from build123d import *

# Parameters (mm, degrees)
SKIZZE1_R                        = 22.5
SEITE1_DEPTH                     = 2
SKIZZE2_R                        = 20.5
LAUFFL_CHE_DEPTH                 = 8
SKIZZE5_R                        = 22.5
SEITE_2_DEPTH                    = 2
BOHRUNG_DEPTH                    = 100
BOHRUNG_DEPTH_BACK               = 34.35416016
SKIZZE7_R                        = 2.5
SKIZZE9_R                        = 10
ZAPFEN_DEPTH                     = 25
SKIZZE10_R                       = 16.5
SEITENTEIL3_DEPTH                = 2
SKIZZE12_R                       = 15
ZAHNFL_CHE_DEPTH                 = 6
SKIZZE14_R                       = 0.56
RIEMENPROFIL_DEPTH               = 6
SKIZZE13_R                       = 16.5
SEITENTEIL4_DEPTH                = 2
F_12_0_12_DURCHMESSER_BOHRUNG1_D = 12


with BuildPart() as part:
    # Skizze1 → Seite1 (new body)
    with BuildSketch(Plane.XY):
        Circle(SKIZZE1_R)
    extrude(amount=SEITE1_DEPTH)

    # Skizze2 → Lauffläche (add)
    with BuildSketch(Plane.XY):
        Circle(SKIZZE2_R)
    extrude(amount=LAUFFL_CHE_DEPTH)

    # Skizze5 → Seite 2 (add)
    with BuildSketch(Plane.XY.offset(8)):
        Circle(SKIZZE5_R)
    extrude(amount=SEITE_2_DEPTH)

    # Skizze7 → Bohrung (cut, two sides: drawn at the far end of the back side and taken through both)
    with BuildSketch(Plane.XY.offset(-BOHRUNG_DEPTH_BACK)):
        Circle(SKIZZE7_R)
    extrude(amount=BOHRUNG_DEPTH + BOHRUNG_DEPTH_BACK, mode=Mode.SUBTRACT)

    # Skizze9 → Zapfen (add)
    with BuildSketch(Plane.XY.offset(10)):
        Circle(SKIZZE9_R)
    extrude(amount=ZAPFEN_DEPTH)

    # Skizze10 → Seitenteil3 (add)
    with BuildSketch(Plane.XY.offset(35)):
        Circle(SKIZZE10_R)
    extrude(amount=SEITENTEIL3_DEPTH)

    # Skizze12 → Zahnfläche (add)
    with BuildSketch(Plane.XY.offset(37)):
        Circle(SKIZZE12_R)
    extrude(amount=ZAHNFL_CHE_DEPTH)

    # Skizze14 → Riemenprofil (cut)
    with BuildSketch(Plane.XY.offset(43)):
        with Locations((0, 15)):
            Circle(SKIZZE14_R)
        with Locations((1.966556951, 14.928861044)):
            Circle(SKIZZE14_R)
        with Locations((3.907004237, 14.6016435)):
            Circle(SKIZZE14_R)
        with Locations((5.788140268, 14.023946153)):
            Circle(SKIZZE14_R)
        with Locations((7.577778284, 13.205653563)):
            Circle(SKIZZE14_R)
        with Locations((9.245297083, 12.160766945)):
            Circle(SKIZZE14_R)
        with Locations((10.762164956, 10.907164596)):
            Circle(SKIZZE14_R)
        with Locations((12.102427872, 9.466296002)):
            Circle(SKIZZE14_R)
        with Locations((13.243153563, 7.862814824)):
            Circle(SKIZZE14_R)
        with Locations((14.164823895, 6.124157069)):
            Circle(SKIZZE14_R)
        with Locations((14.851668833, 4.280071652)):
            Circle(SKIZZE14_R)
        with Locations((15.29193627, 2.362111388)):
            Circle(SKIZZE14_R)
        with Locations((15.478093108, 0.403093108)):
            Circle(SKIZZE14_R)
        with Locations((15.406954151, -1.563463843)):
            Circle(SKIZZE14_R)
        with Locations((15.079736608, -3.503911129)):
            Circle(SKIZZE14_R)
        with Locations((14.502039261, -5.38504716)):
            Circle(SKIZZE14_R)
        with Locations((13.683746671, -7.174685176)):
            Circle(SKIZZE14_R)
        with Locations((12.638860052, -8.842203975)):
            Circle(SKIZZE14_R)
        with Locations((11.385257704, -10.359071848)):
            Circle(SKIZZE14_R)
        with Locations((9.94438911, -11.699334765)):
            Circle(SKIZZE14_R)
        with Locations((8.340907932, -12.840060456)):
            Circle(SKIZZE14_R)
        with Locations((6.602250176, -13.761730787)):
            Circle(SKIZZE14_R)
        with Locations((4.75816476, -14.448575725)):
            Circle(SKIZZE14_R)
        with Locations((2.840204496, -14.888843162)):
            Circle(SKIZZE14_R)
        with Locations((0.881186216, -15.075)):
            Circle(SKIZZE14_R)
        with Locations((-1.085370735, -15.003861044)):
            Circle(SKIZZE14_R)
        with Locations((-3.025818021, -14.6766435)):
            Circle(SKIZZE14_R)
        with Locations((-4.906954052, -14.098946153)):
            Circle(SKIZZE14_R)
        with Locations((-6.696592068, -13.280653563)):
            Circle(SKIZZE14_R)
        with Locations((-8.364110867, -12.235766945)):
            Circle(SKIZZE14_R)
        with Locations((-9.88097874, -10.982164596)):
            Circle(SKIZZE14_R)
        with Locations((-11.221241657, -9.541296002)):
            Circle(SKIZZE14_R)
        with Locations((-12.361967348, -7.937814824)):
            Circle(SKIZZE14_R)
        with Locations((-13.28363768, -6.199157069)):
            Circle(SKIZZE14_R)
        with Locations((-13.970482618, -4.355071652)):
            Circle(SKIZZE14_R)
        with Locations((-14.410750054, -2.437111388)):
            Circle(SKIZZE14_R)
        with Locations((-14.596906892, -0.478093108)):
            Circle(SKIZZE14_R)
        with Locations((-14.525767936, 1.488463843)):
            Circle(SKIZZE14_R)
        with Locations((-14.198550392, 3.428911129)):
            Circle(SKIZZE14_R)
        with Locations((-13.620853045, 5.31004716)):
            Circle(SKIZZE14_R)
        with Locations((-12.802560456, 7.099685176)):
            Circle(SKIZZE14_R)
        with Locations((-11.757673837, 8.767203975)):
            Circle(SKIZZE14_R)
        with Locations((-10.504071489, 10.284071848)):
            Circle(SKIZZE14_R)
        with Locations((-9.063202895, 11.624334765)):
            Circle(SKIZZE14_R)
        with Locations((-7.459721716, 12.765060456)):
            Circle(SKIZZE14_R)
        with Locations((-5.721063961, 13.686730787)):
            Circle(SKIZZE14_R)
        with Locations((-3.876978545, 14.373575725)):
            Circle(SKIZZE14_R)
        with Locations((-1.95901828, 14.813843162)):
            Circle(SKIZZE14_R)
    extrude(amount=-RIEMENPROFIL_DEPTH, mode=Mode.SUBTRACT)

    # Skizze13 → Seitenteil4 (add)
    with BuildSketch(Plane.XY.offset(43)):
        Circle(SKIZZE13_R)
    extrude(amount=SEITENTEIL4_DEPTH)

    # Ø12.0 (12) Durchmesser Bohrung1 (through all)
    with Locations(Plane(origin=(0, 0, 0), x_dir=(-1, 0, 0), z_dir=(0, 0, -1))):
        with Locations((0, 0)):
            Hole(F_12_0_12_DURCHMESSER_BOHRUNG1_D / 2)


solid = part.part
Read the model definition and answer for the solid it produces. Units are mm, in the model's axes. A direction names the side the tool comes from. Round coordinates to 2 decimals unless told otherwise and drop trailing zeros. Write each loop counter-clockwise with the first axis right and the second up, starting at its lowest first coordinate (ties: lowest second). Pieces come first, ordered by that corner, then holes.
1. Which of the six approach directions +Z, -Z, +X, -X, +Y, -Y give full straight-line access (tool end or side, diameter ignored) to faces 1 (the face through (15.24, -6.32, 35.99)), 2 (the face through (-10, -11, 43)), 3 (the face through (14.365, -4.317, 39.958)), 4 (the face through (14.94, 1.33, 39.96))?
2. The part is cut by section A-A, the plane z = 17. Determine the outline of the cut face in (x, y), then the cut area to 3 significant figures.
3. Straight lines are drawn through the part: L1, parallel to Z at x = 3, y = -15; L2, parallel to Y at x = 0, z = 20; L3, parallel to Z at x = 19.5, y = 6. For each, find the intervals that lie inside material, in ascending order.
4. Determine the mould class of faces 5 (the face through (15.24, -6.32, 43.99)), 6 (the face through (-6, 0, 23)), 7 (the face through (9.9, -18.2, 2)) for opening direction Y: pulls with the +Y half, pulls with the -Y half, needs draft (parallel to the pull), parting line crosses it, or undercut.
5. The part is cut by section B-B, the plane z = 3.5. Determine the outline of the cut face in (x, y).
6. Given pin 1 Ø1 at (x, z) = (-1.5, 25.5) entering from -Y; pin 2 Ø1.5 at (y, z) = (3.5, 23) entering from +X; pin 3 Ø1.5 at (x, z) = (2, 23) entering from +Y, each flat-ended and moving along its own axis, determine where each tip first touches the part or whether it passes through.
Values:
1. face 1: +Z
1. face 2: none
1. face 3: +X, -Y
1. face 4: +X, +Y
2. outline: circle Ø20 at (0, 0); hole circle Ø12 at (0, 0)
2. area: 201 mm2
3. L1: z = 0 to 10, 35 to 37, 43 to 45
3. L2: y = -10 to -6, 6 to 10
3. L3: z = 0 to 10
4. face 5: parting line crosses it
4. face 6: undercut
4. face 7: needs draft
5. outline: circle Ø41 at (0, 0); hole circle Ø12 at (0, 0)
6. pin 1: stops at y = -9.95
6. pin 2: stops at x = 9.61
6. pin 3: stops at y = 9.92
